Source: CAD feature listing. Evaluate the final solid. Frame: model axes, mm. Face numbers are marked on the shaded views. A direction names the side the tool comes from. Give positions to 0.01 mm unless a question says otherwise; leave off trailing zeros. Write each loop counter-clockwise with the first axis right and the second up, starting at its lowest first coordinate (ties: lowest second). Pieces come first, ordered by that corner, then holes. Notation, with made-up numbers: M 11.5,24.5 L 48.5,24.5 A23 ccw 48.5,34.5 Z; hole C 42,76 d3. An arc over 180 degrees is marked long. Return JSON: item names as keys, results as strings.
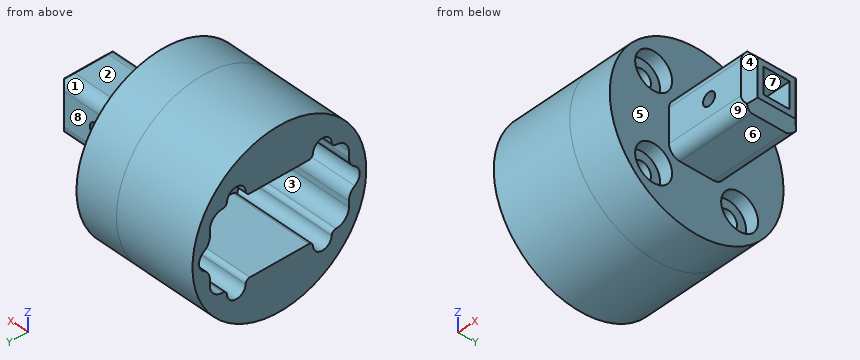
```python
from build123d import *

# Parameters (mm, degrees)
SKETCH_1_R               = 20
EXTRUDE_1_DEPTH          = 10
SKETCH_2_W               = 15
SKETCH_2_H               = 30.5
CUT_EXTRUDE_1_DEPTH      = 4
SKETCH_3_R               = 8.75
CUT_EXTRUDE_2_DEPTH      = 4
EXTRUDE_START            = 19
SKETCH_4_R               = 20
SKETCH_4_W               = 18
SKETCH_4_H               = 32
EXTRUDE_2_DEPTH          = 19
FILLET_1_R               = 3
SKETCH_5_R               = 2.5
CUT_EXTRUDE_3_DEPTH      = 20
FILLET_2_R               = 3
SKETCH_6_R               = 2.15
CUT_EXTRUDE_4_DEPTH      = 43
FILLET_3_R               = 1
SKETCH_7_R               = 4.25
CUT_EXTRUDE_5_DEPTH      = 3
PATTERN_CIRCULAR_1_COUNT = 4
SKETCH_8_W               = 12.7
SKETCH_8_H               = 12.7
EXTRUDE_3_DEPTH          = 20
SKETCH_9_W               = 6
SKETCH_9_H               = 6
CUT_EXTRUDE_6_DEPTH      = 35
SKETCH_10_W              = 3
SKETCH_10_H              = 15
CUT_EXTRUDE_7_DEPTH      = 5
SKETCH_11_R              = 2.5
CUT_EXTRUDE_8_DEPTH      = 5
SKETCH_12_R              = 1.5
CUT_EXTRUDE_9_DEPTH      = 17
CHAMFER_1_SIZE           = 2
FILLET_4_R               = 3
FILLET_5_R               = 2.5


with BuildPart() as part:
    # 草图1 → 凸台-拉伸1 (new body)
    with BuildSketch(Plane(origin=(0, 0, 0), x_dir=(0, 0, -1), z_dir=(1, 0, 0))):
        Circle(SKETCH_1_R)
    extrude(amount=EXTRUDE_1_DEPTH)

    # 草图2 → 切除-拉伸1 (cut)
    with BuildSketch(Plane.ZY):
        Rectangle(SKETCH_2_W, SKETCH_2_H)
    extrude(amount=-CUT_EXTRUDE_1_DEPTH, mode=Mode.SUBTRACT)

    # 草图3 → 切除-拉伸2 (cut)
    with BuildSketch(Plane.ZY.offset(-4)):
        Circle(SKETCH_3_R)
    extrude(amount=CUT_EXTRUDE_2_DEPTH, mode=Mode.SUBTRACT)

    # 草图4 → 凸台-拉伸2 (add)
    with BuildSketch(Plane.ZY.offset(EXTRUDE_START)):
        Circle(SKETCH_4_R)
        Rectangle(SKETCH_4_W, SKETCH_4_H, mode=Mode.SUBTRACT)
    extrude(amount=-EXTRUDE_2_DEPTH)

    # 圆角1
    fillet_1_edges = [part.edges().sort_by_distance(p)[0] for p in [
        (-9.5, 16, 9),
        (-9.5, 16, -9),
        (-9.5, -16, -9),
        (-9.5, -16, 9),
    ]]
    fillet(fillet_1_edges, radius=FILLET_1_R)

    # 草图5 → 切除-拉伸3 (cut)
    with BuildSketch(Plane.ZY.offset(19)):
        with Locations((0, -16)):
            Circle(SKETCH_5_R)
        with Locations((0, 16)):
            Circle(SKETCH_5_R)
    extrude(amount=-CUT_EXTRUDE_3_DEPTH, mode=Mode.SUBTRACT)

    # 圆角2
    # the kernel refuses this fillet: 3 mm, written as the material it takes off along each edge
    with BuildSketch(Plane(origin=(-24.274430572, -16, 2.5), x_dir=(0, -0.9586814917396833, -0.2844816292764363), z_dir=(1, 0, 0))) as fillet_2_piece_1:
        with BuildLine():
            CenterArc((2.275853034, -2.876044475), FILLET_2_R, 106.527865575, 56.944268849)
            Line((-0.600191441, -2.022599587), (0, 0))
            ThreePointArc((0, 0), (0.711204073, -0.103296271), (1.422408146, 0))
        make_face()
    extrude(amount=24.274430572, mode=Mode.SUBTRACT)
    with BuildSketch(Plane(origin=(0, -16, -2.5), x_dir=(0, 0, -1), z_dir=(-1, 0, 0))) as fillet_2_piece_2:
        with BuildLine():
            CenterArc((2.109772229, 3), FILLET_2_R, 213.055731151, 56.944268849)
            ThreePointArc((-0.404648987, 1.363636364), (-0.103296271, 0.711204073), (0, 0))
            Line((0, 0), (2.109772229, 0))
        make_face()
    extrude(amount=24.274430572, mode=Mode.SUBTRACT)
    with BuildSketch(Plane(origin=(0, 16, -2.5), x_dir=(0, 0.9586814917396834, 0.2844816292764354), z_dir=(-1, 0, 0))) as fillet_2_piece_3:
        with BuildLine():
            CenterArc((2.275853034, 2.876044475), FILLET_2_R, 196.527865575, 56.944268849)
            Line((-0.600191441, 2.022599587), (0, 0))
            ThreePointArc((0, 0), (0.711204073, 0.103296271), (1.422408146, 0))
        make_face()
    extrude(amount=24.274430572, mode=Mode.SUBTRACT)
    with BuildSketch(Plane(origin=(-24.274430572, 16, 2.5), x_dir=(0, 0, 1), z_dir=(1, 0, 0))) as fillet_2_piece_4:
        with BuildLine():
            CenterArc((2.109772229, -3), FILLET_2_R, 90, 56.944268849)
            ThreePointArc((-0.404648987, -1.363636364), (-0.103296271, -0.711204073), (0, 0))
            Line((0, 0), (2.109772229, 0))
        make_face()
    extrude(amount=24.274430572, mode=Mode.SUBTRACT)

    # 草图6 → 切除-拉伸4 (cut)
    with BuildSketch(Plane(origin=(10, 0, 0), x_dir=(0, 0, -1), z_dir=(1, 0, 0))):
        with Locations((9.899494937, -9.899494937)):
            Circle(SKETCH_6_R)
        with Locations((-9.899494937, -9.899494937)):
            Circle(SKETCH_6_R)
        with Locations((-9.899494937, 9.899494937)):
            Circle(SKETCH_6_R)
        with Locations((9.899494937, 9.899494937)):
            Circle(SKETCH_6_R)
    extrude(amount=-CUT_EXTRUDE_4_DEPTH, mode=Mode.SUBTRACT)

    # 圆角3
    # the kernel refuses this fillet: 1 mm, written as the material it takes off along each edge
    with BuildSketch(Plane(origin=(-21.98900269, -7.946699797, 9), x_dir=(0, 0.1985408891964352, 0.9800926054802622), z_dir=(1, 0, 0)), Plane(origin=(-21.98900269, 7.946699797, -9), x_dir=(0, -0.19854088919647347, -0.9800926054802545), z_dir=(1, 0, 0))) as fillet_3_piece_1:
        with BuildLine():
            CenterArc((1.217468306, -0.973258884), FILLET_3_R, 103.280057781, 88.171589383)
            Line((0.237375701, -1.171799774), (0, 0))
            ThreePointArc((0, 0), (0.493878653, -0.057493399), (0.987757305, 0))
        make_face()
    extrude(amount=21.98900269, mode=Mode.SUBTRACT)
    with BuildSketch(Plane(origin=(-21.959087911, -11.852290077, 9), x_dir=(0, -0.999999983485678, -0.00018173784322620402), z_dir=(1, 0, 0)), Plane(origin=(-21.959087911, 11.852290077, -9), x_dir=(0, 0.9999999834856781, 0.00018173784322619477), z_dir=(1, 0, 0))) as fillet_3_piece_2:
        with BuildLine():
            CenterArc((1.195428513, -0.999930456), FILLET_3_R, 90.675724778, 87.490671362)
            Line((0.195940547, -0.967933494), (0.09599175, -0.964733798))
            ThreePointArc((0.09599175, -0.964733798), (0.056286672, -0.492404834), (-0.090835283, -0.041820466))
            Line((-0.090835283, -0.041820466), (1.8174e-05, 0.099999998))
            ThreePointArc((1.8174e-05, 0.099999998), (1.147728078, 0.099791416), (1.182455829, 0.099993046))
            Line((1.182455829, 0.099993046), (1.183635164, 0))
        make_face()
    extrude(amount=21.959087911, mode=Mode.SUBTRACT)
    with BuildSketch(Plane(origin=(-21.959087911, -11.852290077, -9), x_dir=(0, -0.19858553154825268, -0.98008356105982), z_dir=(1, 0, 0)), Plane(origin=(-21.959087911, 11.852290077, 9), x_dir=(0, 0.19858553154822475, 0.9800835610598256), z_dir=(1, 0, 0))) as fillet_3_piece_3:
        with BuildLine():
            CenterArc((1.217233349, -0.973269347), FILLET_3_R, 103.277447997, 87.490671362)
            Line((0.234841987, -1.160104066), (0.136602851, -1.178787538))
            ThreePointArc((0.136602851, -1.178787538), (0.129910229, -1.144710182), (-0.098008356, -0.019858553))
            Line((-0.098008356, -0.019858553), (0.022966667, 0.097326935))
            ThreePointArc((0.022966667, 0.097326935), (0.49378334, 0.042529095), (0.964600013, 0.097326935))
            Line((0.964600013, 0.097326935), (0.987566679, 0))
        make_face()
    extrude(amount=21.959087911, mode=Mode.SUBTRACT)
    with BuildSketch(Plane(origin=(-21.98900269, -7.946699797, -9), x_dir=(0, 1, 0), z_dir=(1, 0, 0)), Plane(origin=(-21.98900269, 7.946699797, 9), x_dir=(0, -1, 0), z_dir=(1, 0, 0))) as fillet_3_piece_4:
        with BuildLine():
            CenterArc((1.195601076, -1), FILLET_3_R, 90, 88.171589383)
            ThreePointArc((0.196110214, -0.968093631), (0.154403962, -0.472632025), (0, 0))
            Line((0, 0), (1.195601076, 0))
        make_face()
    extrude(amount=21.98900269, mode=Mode.SUBTRACT)

    # 草图7 → 切除-拉伸5 (cut)
    with BuildSketch(Plane(origin=(10, 0, 0), x_dir=(0, 0, -1), z_dir=(1, 0, 0))):
        with Locations((9.899494937, -9.899494937)):
            Circle(SKETCH_7_R)
    cut_extrude_5 = extrude(amount=-CUT_EXTRUDE_5_DEPTH, mode=Mode.SUBTRACT)

    # 阵列(圆周)1: 切除-拉伸5 ×4 about axis
    pattern_circular_1_axis = Axis((0, 0, 0), (1, 0, 0))
    for i in range(1, PATTERN_CIRCULAR_1_COUNT):
        add(cut_extrude_5.rotate(pattern_circular_1_axis, i * 360 / PATTERN_CIRCULAR_1_COUNT), mode=Mode.SUBTRACT)

    # 草图8 → 凸台-拉伸3 (add)
    with BuildSketch(Plane(origin=(10, 0, 0), x_dir=(0, 0, -1), z_dir=(1, 0, 0))):
        Rectangle(SKETCH_8_W, SKETCH_8_H)
    extrude(amount=EXTRUDE_3_DEPTH)

    # 草图9 → 切除-拉伸6 (cut)
    with BuildSketch(Plane(origin=(30, 0, 0), x_dir=(0, 0, -1), z_dir=(1, 0, 0))):
        Rectangle(SKETCH_9_W, SKETCH_9_H)
    extrude(amount=-CUT_EXTRUDE_6_DEPTH, mode=Mode.SUBTRACT)

    # 草图10 → 切除-拉伸7 (cut)
    with BuildSketch(Plane.ZY.offset(-1)):
        with Locations((0, 10.5)):
            Rectangle(SKETCH_10_W, SKETCH_10_H)
    extrude(amount=-CUT_EXTRUDE_7_DEPTH, mode=Mode.SUBTRACT)

    # 草图11 → 切除-拉伸8 (cut)
    with BuildSketch(Plane.ZY.offset(-1)):
        with Locations((0, 16)):
            Circle(SKETCH_11_R)
    extrude(amount=-CUT_EXTRUDE_8_DEPTH, mode=Mode.SUBTRACT)

    # 草图12 → 切除-拉伸9 (cut)
    with BuildSketch(Plane.XZ.offset(6.35)):
        with Locations(Location((20, 0, 0), (0, 0, 270))):
            Circle(SKETCH_12_R)
    extrude(amount=-CUT_EXTRUDE_9_DEPTH, mode=Mode.SUBTRACT)

    # 倒角1
    chamfer_1_edges = [part.edges().sort_by_distance(p)[0] for p in [
        (30, 0, 6.35),
        (30, -6.35, 0),
        (30, 0, -6.35),
        (30, 6.35, 0),
    ]]
    chamfer(chamfer_1_edges, length=CHAMFER_1_SIZE)

    # 圆角4
    fillet_4_edges = [part.edges().sort_by_distance(p)[0] for p in [
        (6, 3, 0),
    ]]
    fillet(fillet_4_edges, radius=FILLET_4_R)

    # 圆角5
    fillet_5_edges = [part.edges().sort_by_distance(p)[0] for p in [
        (19, -6.35, 6.35),
        (19, 6.35, 6.35),
        (19, 6.35, -6.35),
        (19, -6.35, -6.35),
    ]]
    fillet(fillet_5_edges, radius=FILLET_5_R)


solid = part.part
```
1) Cut plane B-B, the plane y = 0. Return the cut outline in (x, z).
Numbers:
{"outline": "M -19,-20 L 10,-20 L 10,-6.35 L 28,-6.35 L 30,-4.35 L 30,-3 L 4,-3 L 4,-8.75 L 0,-8.75 L 0,-9 L -19,-9 Z; M -19,9 L 0,9 L 0,8.75 L 4,8.75 L 4,3 L 30,3 L 30,4.35 L 28,6.35 L 10,6.35 L 10,20 L -19,20 Z"}
2) Contact query for flat-ended pins moving along their axis: pin 1 Ø2 at (x, y) = (0.5, -13.5) entering from -Z; pin 2 Ø2.5 at (x, y) = (21.5, -0.5) entering from -Z; pin 3 Ø4 at (y, z) = (-7.5, -4.5) entering from +X. Output: stop coordinate, or through.
Numbers:
{"pin 1": "stops at z = -15.61", "pin 2": "stops at z = -6.35", "pin 3": "stops at x = 28.85"}
3) Line query: line 1 (Y direction, x = -6, z = 0); line 2 (X direction, y = 4, z = 0); line 3 (Z direction, x = 25, y = -2.5). Output: solid intervals per line, ascending. Write a range as [from, to].
Numbers:
{"line 1": "y = [-20, -18.5], [18.5, 20]", "line 2": "x = [6.76, 18.5], [21.5, 30]", "line 3": "z = [-6.35, -3], [3, 6.35]"}
4) Cut plane D-D, the plane x = 12. Return the cut outline in (y, z).
Numbers:
{"outline": "M -6.35,-3.85 A2.5 ccw -3.85,-6.35 L 3.85,-6.35 A2.5 ccw 6.35,-3.85 L 6.35,3.85 A2.5 ccw 3.85,6.35 L -3.85,6.35 A2.5 ccw -6.35,3.85 Z; hole M -3,-3 L 3,-3 L 3,3 L -3,3 Z"}
5) Cut plane C-C, the plane x = 20. Return the cut outline in (y, z).
Numbers:
{"outline": "M -6.35,-3.85 A2.5 ccw -3.85,-6.35 L 3.85,-6.35 A2.5 ccw 6.35,-3.85 L 6.35,-1.5 L 3,-1.5 L 3,-3 L -3,-3 L -3,-1.5 L -6.35,-1.5 Z; M -6.35,1.5 L -3,1.5 L -3,3 L 3,3 L 3,1.5 L 6.35,1.5 L 6.35,3.85 A2.5 ccw 3.85,6.35 L -3.85,6.35 A2.5 ccw -6.35,3.85 Z"}
6) Set-up query: the marked faces 5, 6, 7, 8 and 9. Return all of +Z, -Z, +X, -X, +Y, -Y with unobstructed straight access to the full face (end or side cutting, diameter ignored); none if empty.
Numbers:
{"face 5": "+X", "face 6": "-Z, +X, +Y, -Y", "face 7": "+X, -X", "face 8": "+Z, -Z, +X, +Y", "face 9": "-Z, +X, -Y"}
7) Draft query along Y for the marked faces 1, 2, 3 and 4. Return one class per face: released by +Y, released by -Y, zero draft, split by the parting line, or undercut.
Numbers:
{"face 1": "released by +Y", "face 2": "zero draft", "face 3": "undercut", "face 4": "released by -Y"}
